Part print with two shaded views. Sizes in mm from the minimum x, y, z corner. A direction names the side the tool comes from. Round coordinates to 2 decimals unless told otherwise and drop trailing zeros. Order: outer loops, then holes, each group sorted by start corner. A loop starts at its lowest first (then second) coordinate and runs counter-clockwise, first axis right, second up. Notation, with made-up numbers: (82.5, -12.5) - (101.5, -12.5) arc R23 cw to (101.5, 21.5) - close; hole circle Ø9 at (46, 21). An arc over 180 degrees is marked (long way). Use one line per item in the form item = value.
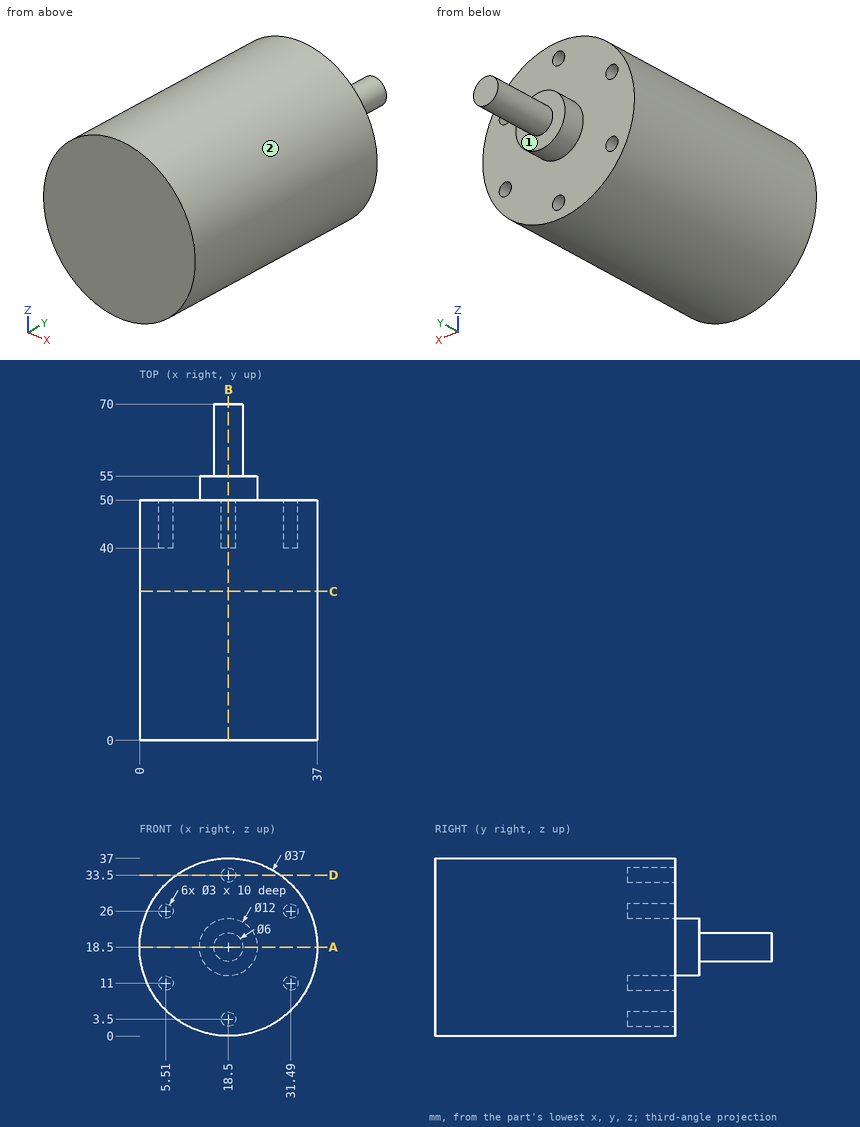
(1) Probe probe 1 along X at (y, z) = (45, 11); probe 2 along Y at (x, z) = (28.5, 12); probe 3 along Y at (x, z) = (16, 16.5). List the from-to ranges inside material, lowest first. Write a range as [from, to].
Report:
probe_1 = [1.59, 4.01], [7.01, 29.99], [32.99, 35.41]
probe_2 = [0, 50]
probe_3 = [0, 55]
(2) Tool access for the marked faces 1 and 2: list every direction of +Z, -Z, +X, -X, +Y, -Y with a clear straight run to the whole face (end or side of a thin tool).
Report:
face_1 = +Y
face_2 = +Y, -Y
(3) Slice it at C-C on y = 31. Give the cut face in (x, z), then the cut area to 3 significant figures.
Report:
outline = circle Ø37 at (18.5, 18.5)
area = 1,080 mm2
(4) Slice it at B-B on x = 18.5. Give the cut face in (y, z).
Report:
outline = (0, 0) - (50, 0) - (50, 2) - (40, 2) - (40, 5) - (50, 5) - (50, 12.5) - (55, 12.5) - (55, 15.5) - (70, 15.5) - (70, 21.5) - (55, 21.5) - (55, 24.5) - (50, 24.5) - (50, 32) - (40, 32) - (40, 35) - (50, 35) - (50, 37) - (0, 37) - close
(5) Pin check, flat tips, straight feed: pin 1 (2 mm diameter, centred on x = 10.5, z = 13, fed in from +Y); pin 2 (1.8 mm diameter, centred on x = 18.5, z = 3.5, fed in from -Y); pin 3 (0.9 mm diameter, centred on x = 31, z = 25.5, fed in from +Y); pin 4 (2 mm diameter, centred on y = 49, z = 9.5, fed in from +X). Stop position of each tip, or through.
Report:
pin_1 = 50
pin_2 = 0
pin_3 = 40
pin_4 = 35.18
(6) Slice it at A-A on z = 18.5. Give the cut face in (x, y).
Report:
outline = (0, 0) - (37, 0) - (37, 50) - (24.5, 50) - (24.5, 55) - (21.5, 55) - (21.5, 70) - (15.5, 70) - (15.5, 55) - (12.5, 55) - (12.5, 50) - (0, 50) - close
(7) Slice it at D-D on z = 33.5. Give the cut face in (x, y), then the cut area to 3 significant figures.
Report:
outline = (7.67, 0) - (29.33, 0) - (29.33, 50) - (20, 50) - (20, 40) - (17, 40) - (17, 50) - (7.67, 50) - close
area = 1,050 mm2
